from build123d import *

# Parameters (mm, degrees)
BOSS_EXTRUDE1_DEPTH = 300
SKETCH2_R           = 2.25
CUT_EXTRUDE1_DEPTH  = 10
SKETCH3_R           = 2.25
CUT_EXTRUDE2_DEPTH  = 10
SKETCH5_R           = 2.25
CUT_EXTRUDE3_DEPTH  = 10


with BuildPart() as part:
    # Sketch1 → Boss-Extrude1 (new body)
    with BuildSketch(Plane(origin=(0, 0, 0), x_dir=(1, 0, 0), z_dir=(0, 1, 0))):
        Polygon((0, 0), (12.7, 0), (12.7, 2), (2, 2), (2, 12.7), (0, 12.7), align=None)
    extrude(amount=BOSS_EXTRUDE1_DEPTH)

    # Sketch2 → Cut-Extrude1 (cut)
    with BuildSketch(Plane(origin=(0, 0, -2), x_dir=(-1, 0, 0), z_dir=(0, 0, -1))):
        with Locations((-7.35, 275)):
            Circle(SKETCH2_R)
        with Locations((-7.35, 175)):
            Circle(SKETCH2_R)
        with Locations((-7.35, 75)):
            Circle(SKETCH2_R)
    extrude(amount=-CUT_EXTRUDE1_DEPTH, mode=Mode.SUBTRACT)

    # Sketch3 → Cut-Extrude2 (cut)
    with BuildSketch(Plane(origin=(2, 0, 0), x_dir=(0, 0, -1), z_dir=(1, 0, 0))):
        with Locations((7.35, 225)):
            Circle(SKETCH3_R)
        with Locations((7.35, 125)):
            Circle(SKETCH3_R)
        with Locations((7.35, 25)):
            Circle(SKETCH3_R)
    extrude(amount=-CUT_EXTRUDE2_DEPTH, mode=Mode.SUBTRACT)

    # Sketch5 → Cut-Extrude3 (cut)
    with BuildSketch(Plane.ZY):
        with Locations((-7.94, 253.6)):
            Circle(SKETCH5_R)
    extrude(amount=-CUT_EXTRUDE3_DEPTH, mode=Mode.SUBTRACT)


solid = part.part
The model under review builds one solid part; all positions refer to its coordinate system, in mm. A direction names the side the tool comes from. Round coordinates to 2 decimals unless told otherwise and drop trailing zeros. Order: outer loops, then holes, each group sorted by start corner. A loop starts at its lowest first (then second) coordinate and runs counter-clockwise, first axis right, second up. Notation, with made-up numbers: (-24.5, 83) -> (0.5, 83) arc R21 cw to (0.5, 88) -> close; hole circle Ø1 at (36.5, -24). An arc over 180 degrees is marked (long way). Use CSV: the item, a comma, the result in double quotes. Start each with the question number.
(1) Consider section A-A on x = 7.35. Write out the cut boundary in (y, z).
(2) Consider section B-B on y = 169. Write out the cut boundary in (x, z).
(3) Wall thickness on probe 1 along Y at (x, z) = (7.35, -1.05); probe 2 along Z at (x, y) = (1, 225); probe 3 along Y at (x, z) = (1.6, -7.94): over which ranges is each line inside the solid? List them lowest first. Write a range as from..to.
(4) Insertion check: pin 1 (3 mm diameter, centred on x = 10.5, y = 33.5, fed in from -Z); pin 2 (6 mm diameter, centred on x = 3.5, y = 110, fed in from +Z); pin 3 (5 mm diameter, centred on y = 25, z = -7.35, fed in from +X). Each pin has a flat end and moves straight along its axis. Give the tip position at first contact, or say it passes through.
(5) Tool access review of faces 1 (the face through (0, 148, -6)), 2 (the face through (2, 148, -7)): name each direction out of +Z, -Z, +X, -X, +Y, -Y from which nothing blocks a thin tool from reaching the whole face with its end or side.
Responses:
1,outline,"(0, -2) -> (72.75, -2) -> (72.75, 0) -> (0, 0) -> close; (77.25, -2) -> (172.75, -2) -> (172.75, 0) -> (77.25, 0) -> close; (177.25, -2) -> (272.75, -2) -> (272.75, 0) -> (177.25, 0) -> close; (277.25, -2) -> (300, -2) -> (300, 0) -> (277.25, 0) -> close"
2,outline,"(0, -12.7) -> (2, -12.7) -> (2, -2) -> (12.7, -2) -> (12.7, 0) -> (0, 0) -> close"
3,probe 1,"0..72.75, 77.25..172.75, 177.25..272.75, 277.25..300"
3,probe 2,"-12.7..-9.6, -5.1..0"
3,probe 3,"0..22.83, 27.17..122.83, 127.17..222.83, 227.17..251.35, 255.85..300"
4,pin 1,"z = -2"
4,pin 2,"z = 0"
4,pin 3,"x = 2"
5,face 1,"+Z, -Z, -X, +Y, -Y"
5,face 2,"-Z, +X, +Y, -Y"
